```python
from build123d import *

# Parameters (mm, degrees)
SKETCH_1_W               = 23.3
SKETCH_1_H               = 19
EXTRUDE_1_DEPTH          = 70
SKETCH_2_W               = 10
SKETCH_2_H               = 9
EXTRUDE_2_DEPTH          = 9
SKETCH_3_R               = 2
CUT_EXTRUDE_1_DEPTH      = 6
CUT_EXTRUDE_1_DEPTH_BACK = 15
SKETCH_4_W               = 12
SKETCH_4_H               = 12
EXTRUDE_3_DEPTH          = 110
SKETCH_5_W               = 14.5
SKETCH_5_H               = 14.5
EXTRUDE_4_DEPTH          = 6
SKETCH_6_R               = 4.5
EXTRUDE_5_DEPTH          = 10.5
CUT_EXTRUDE_3_DEPTH      = 10.5
SKETCH_8_R               = 2
CUT_EXTRUDE_4_DEPTH      = 13.5


with BuildPart() as part:
    # 草图1 → 凸台-拉伸1 (new body)
    with BuildSketch(Plane(origin=(0, 0, 0), x_dir=(1, 0, 0), z_dir=(0, 1, 0))):
        Rectangle(SKETCH_1_W, SKETCH_1_H)
    extrude(amount=EXTRUDE_1_DEPTH)

    # 草图2 → 凸台-拉伸2 (add)
    with BuildSketch(Plane(origin=(0, 70, 0), x_dir=(1, 0, 0), z_dir=(0, 1, 0))):
        Rectangle(SKETCH_2_W, SKETCH_2_H)
    extrude(amount=EXTRUDE_2_DEPTH)

    # 草图3 → 切除-拉伸1 (cut, two sides)
    with BuildSketch(Plane.XY.offset(4.5)) as cut_extrude_1_sk:
        with Locations((0, 74.5)):
            Circle(SKETCH_3_R)
    extrude(amount=CUT_EXTRUDE_1_DEPTH, mode=Mode.SUBTRACT)
    extrude(cut_extrude_1_sk.sketch, amount=-CUT_EXTRUDE_1_DEPTH_BACK, mode=Mode.SUBTRACT)

    # 草图4 → 凸台-拉伸3 (add)
    with BuildSketch(Plane.XZ):
        Rectangle(SKETCH_4_W, SKETCH_4_H)
    extrude(amount=EXTRUDE_3_DEPTH)

    # 草图5 → 凸台-拉伸4 (add)
    with BuildSketch(Plane.XZ.offset(110)):
        Rectangle(SKETCH_5_W, SKETCH_5_H)
    extrude(amount=EXTRUDE_4_DEPTH)

    # 草图6 → 凸台-拉伸5 (add)
    with BuildSketch(Plane.XZ.offset(116)):
        Circle(SKETCH_6_R)
    extrude(amount=EXTRUDE_5_DEPTH)

    # 草图7 → 切除-拉伸3 (cut)
    with BuildSketch(Plane.XZ.offset(126.5)):
        with BuildLine():
            Line((-3.354101966, -3), (3.354101966, -3))
            ThreePointArc((3.354101966, -3), (0, -4.5), (-3.354101966, -3))
        make_face()
        with BuildLine():
            Line((-3.354101966, 3), (3.354101966, 3))
            ThreePointArc((3.354101966, 3), (0, 4.5), (-3.354101966, 3))
        make_face()
    extrude(amount=-CUT_EXTRUDE_3_DEPTH, mode=Mode.SUBTRACT)

    # 草图8 → 切除-拉伸4 (cut, through all)
    with BuildSketch(Plane(origin=(0, 0, -3), x_dir=(-1, 0, 0), z_dir=(0, 0, -1))):
        with Locations((0, -122.5)):
            Circle(SKETCH_8_R)
    extrude(amount=-CUT_EXTRUDE_4_DEPTH, mode=Mode.SUBTRACT)


solid = part.part
```
Check sheet for the modelled part. Datum: model origin and axes. Units: mm. A direction names the side the tool comes from. Give positions to 0.01 mm unless a question says otherwise; leave off trailing zeros. Loops run counter-clockwise (first coordinate to the right, second up) from the corner with the lowest first, then second, coordinate; pieces in that order, holes last. Notation, with made-up numbers: M 10,54 L 44,54 A37 ccw 44,90 Z; hole C 88,44.5 d2. An arc over 180 degrees is marked long. Answer in a Markdown table with one row per item.
1) Cross-section at B-B (x = 0). Enter the section's corners in (y, z).
Solutions:
| item | result |
|---|---|
| outline | M -126.5,-3 L -124.5,-3 L -124.5,3 L -126.5,3 Z; M -120.5,-3 L -116,-3 L -116,-7.25 L -110,-7.25 L -110,-6 L 0,-6 L 0,-9.5 L 70,-9.5 L 70,-4.5 L 72.5,-4.5 L 72.5,4.5 L 70,4.5 L 70,9.5 L 0,9.5 L 0,6 L -110,6 L -110,7.25 L -116,7.25 L -116,3 L -120.5,3 Z; M 76.5,-4.5 L 79,-4.5 L 79,4.5 L 76.5,4.5 Z |
2) Depth check by flat-ended pin: pin 1 (4 mm diameter, centred on x = -3, y = -100.5, fed in from +Z); pin 2 (10 mm diameter, centred on y = 76.5, z = 0.5, fed in from +X); pin 3 (7 mm diameter, centred on y = 74, z = 1.5, fed in from -X). Enter the tip coordinate at first touch or a pass-through.
Solutions:
| item | result |
|---|---|
| pin 1 | stops at z = 6 |
| pin 2 | stops at x = 5 |
| pin 3 | stops at x = -5 |
3) Thickness scan on line 1 (Y direction, x = 0, z = -0.25); line 2 (Y direction, x = -7, z = -3.75); line 3 (Y direction, x = 9.5, z = -6.5). Record the ranges inside material, lowest first.
Solutions:
| item | result |
|---|---|
| line 1 | y = -126.5 to -124.5, -120.5 to 72.5, 76.5 to 79 |
| line 2 | y = -116 to -110, 0 to 70 |
| line 3 | y = 0 to 70 |
4) Tool access check on faces 4 (the face through (0, 72, -4.5)), 5 (the face through (-4.5, -121.2, 0)), 6 (the face through (6, -54, 0)), 7 (the face through (5, 74, 0)), 8 (the face through (0, -120, -3)). Record the directions out of +Z, -Z, +X, -X, +Y, -Y that give a thin tool (end or side, any length) a straight path to the whole face; none if there is none.
Solutions:
| item | result |
|---|---|
| face 4 | -Z, +X, -X, +Y |
| face 5 | -X, -Y |
| face 6 | +Z, -Z, +X |
| face 7 | +Z, -Z, +X, +Y |
| face 8 | -Z, +X, -X, -Y |
5) Cross-section at C-C (y = 74.5). Enter the section's corners in (x, z), plus the area to 3 significant figures.
Solutions:
| item | result |
|---|---|
| outline | M -5,-4.5 L -2,-4.5 L -2,4.5 L -5,4.5 Z; M 2,-4.5 L 5,-4.5 L 5,4.5 L 2,4.5 Z |
| area | 54.0 mm^2 |
6) Mould release check, pull along Y, two halves, no side actions. Record for faces 1 (the face through (-1.075, -120.814, -0.042)), 2 (the face through (7.25, -113, 0)), 3 (the face through (-0.1, -116, 3.3)): released by +Y, released by -Y, zero draft, split by the parting line, or undercut.
Solutions:
| item | result |
|---|---|
| face 1 | undercut |
| face 2 | zero draft |
| face 3 | released by -Y |
7) Cross-section at D-D (y = -50). Enter the section's corners in (x, z).
Solutions:
| item | result |
|---|---|
| outline | M -6,-6 L 6,-6 L 6,6 L -6,6 Z |
8) Cross-section at A-A (y = -122.5). Enter the section's corners in (x, z), plus the area to 3 significant figures.
Solutions:
| item | result |
|---|---|
| outline | M -3.35,-3 L -2,-3 L -2,3 L -3.35,3 A4.5 ccw Z; M 2,-3 L 3.35,-3 A4.5 ccw 3.35,3 L 2,3 Z |
| area | 25.7 mm^2 |
